from build123d import *

# Parameters (mm, degrees)
BOSS_EXTRUDE1_DEPTH = 7
FILLET1_R           = 3
FILLET2_R           = 5
SKETCH2_W           = 5
SKETCH2_H           = 40
BOSS_EXTRUDE2_DEPTH = 22
SKETCH4_R           = 1.5
CUT_EXTRUDE1_DEPTH  = 3
SKETCH5_R           = 1.5
CUT_EXTRUDE2_DEPTH  = 5
FILLET3_R           = 1


with BuildPart() as part:
    # Sketch1 → Boss-Extrude1 (new body)
    with BuildSketch(Plane(origin=(0, 0, 0), x_dir=(0, 0, -1), z_dir=(1, 0, 0))):
        Polygon((-21.785617828, -17.377868865), (35.214382172, -17.377868865), (35.214382172, 22.622131135), (23.214382172, 22.622131135), (23.214382172, 16.622131135), (1.187686697, 3.773991719), (3.455005417, -0.113072189), (-20.299274017, -13.968908814), (-22.566592737, -10.081844907), (-42.433808264, -21.670362811), (-38.937098948, -27.665079148), align=None)
        Polygon((23.234116709, 8.569586546), (23.234116709, -10.417868865), (4.764740561, -10.417868865), (4.764740561, -1.399885987), (6.011600394, -1.399885987), align=None, mode=Mode.SUBTRACT)
        Polygon((-39.613886954, -22.304550046), (-34.634489281, -19.42911985), (-33.384302239, -21.59407536), (-38.363699913, -24.469505556), align=None, mode=Mode.SUBTRACT)
        Polygon((-9.735540794, -10.497868865), (-2.235259439, -10.497868865), (-2.235259439, -6.248372162), align=None, mode=Mode.SUBTRACT)
        Polygon((16.699385829, 10.182861543), (17.951839541, 8.019216032), (22.7118599, 10.774614335), (21.459406188, 12.938259845), align=None, mode=Mode.SUBTRACT)
    extrude(amount=-BOSS_EXTRUDE1_DEPTH)

    # Fillet1
    # the kernel refuses this fillet: 3 mm, written as the material it adds along each edge
    with BuildSketch(Plane(origin=(0, -10.417868865, -4.764740561), x_dir=(0, 0, -1), z_dir=(-1, 0, 0))) as fillet1_piece_1:
        with BuildLine():
            CenterArc((FILLET1_R, -FILLET1_R), FILLET1_R, 90, 90)
            Line((0, -FILLET1_R), (-FILLET1_R * 0.02, -FILLET1_R))
            Line((-FILLET1_R * 0.02, -FILLET1_R), (-FILLET1_R * 0.02, FILLET1_R * 0.02))
            Line((-FILLET1_R * 0.02, FILLET1_R * 0.02), (FILLET1_R, FILLET1_R * 0.02))
            Line((FILLET1_R, FILLET1_R * 0.02), (FILLET1_R, 0))
        make_face()
    extrude(amount=7)
    with BuildSketch(Plane(origin=(0, -1.399885987, -4.764740561), x_dir=(0, -1, 0), z_dir=(-1, 0, 0))) as fillet1_piece_2:
        with BuildLine():
            CenterArc((2.434440295, -3), FILLET1_R, 90, 54.240794128)
            Line((0, -1.246859832), (-0.048688806, -1.211797029))
            ThreePointArc((-0.048688806, -1.211797029), (-0.06, -0.623429916), (-0.06, 0))
            Line((-0.06, 0), (0, 0.06))
            Line((0, 0.06), (2.434440295, 0.06))
            Line((2.434440295, 0.06), (2.434440295, 0))
        make_face()
    extrude(amount=7)

    # Fillet2
    fillet2_edges = [part.edges().sort_by_distance(p)[0] for p in [
        (-3.5, -10.417868865, -23.234116709),
    ]]
    fillet(fillet2_edges, radius=FILLET2_R)

    # Sketch2 → Boss-Extrude2 (add)
    with BuildSketch(Plane.ZY.offset(7)):
        with Locations((-32.714382172, 2.622131135)):
            Rectangle(SKETCH2_W, SKETCH2_H)
    extrude(amount=BOSS_EXTRUDE2_DEPTH)

    # Sketch4 → Cut-Extrude1 (cut)
    with BuildSketch(Plane(origin=(0, 2.299007828, 1.341007921), x_dir=(1, 0, 0), z_dir=(0, 0.8637919794098133, 0.5038486045502921))):
        with Locations(Location((-3.5, 22.427434704, 0), (0, 0, 270))):
            Circle(SKETCH4_R)
        with Locations(Location((-3.5, -42.572565296, 0), (0, 0, 270))):
            Circle(SKETCH4_R)
    extrude(amount=-CUT_EXTRUDE1_DEPTH, mode=Mode.SUBTRACT)

    # Sketch5 → Cut-Extrude2 (cut)
    with BuildSketch(Plane.XY.offset(-30.214382172)):
        with Locations((-21, 7.622131135)):
            Circle(SKETCH5_R)
        with Locations((-21, -12.377868865)):
            Circle(SKETCH5_R)
    extrude(amount=-CUT_EXTRUDE2_DEPTH, mode=Mode.SUBTRACT)

    # Fillet3
    fillet3_edges = [part.edges().sort_by_distance(p)[0] for p in [
        (-29, 2.622131135, -35.214382172),
        (-29, -17.377868865, -32.714382172),
        (-29, 2.622131135, -30.214382172),
        (-29, 22.622131135, -32.714382172),
    ]]
    fillet(fillet3_edges, radius=FILLET3_R)


solid = part.part
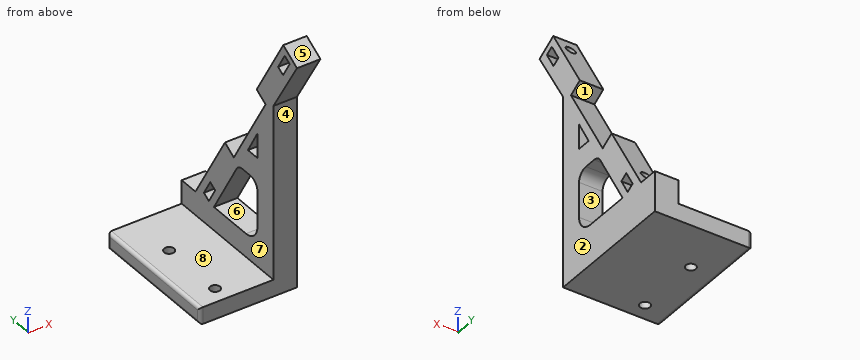
The listing builds one solid part. Answer for the finished solid, in the listing's coordinates (mm). Face numbers are marked on the shaded views. A direction names the side the tool comes from. Coordinates: 2 decimals unless noted, no trailing zeros. Loops run counter-clockwise (first coordinate to the right, second up) from the corner with the lowest first, then second, coordinate; pieces in that order, holes last.
1) Find the intervals of material crossed by L1, parallel to Y at x = -21, z = -33.8; L2, parallel to Y at x = -6.5, z = -17; L3, parallel to Z at x = -9, y = 3, in increasing order.
2) A tool of negligible diameter and unlimited length cuts with its end or side. For the marked faces 1, 2, 3, 4 and 5, from which of +Z, -Z, +X, -X, +Y, -Y can it reach the whole face along a straight path? Write none if from no direction.
3) Determine the mould class of the marked faces 6, 7 and 8 for opening direction Z: pulls with the +Z half, pulls with the -Z half, needs draft (parallel to the pull), parting line crosses it, or undercut.
4) Find section B-B on z = 5. Write down the section's boundary in (x, y).
5) Find section A-A on x = -21. Write down the section's boundary in (y, z).
6) Find section D-D on y = 5. Write down the section's boundary in (x, z).
7) Flat-ended cylindrical pins translate along their axes: pin 1 Ø1.5 at (x, z) = (-8, 14) entering from -Y; pin 2 Ø1.3 at (x, y) = (-4.5, -9) entering from +Z (3 decimals); pin 3 Ø7.5 at (x, z) = (-4, 7.5) entering from +Y; pin 4 Ø1.8 at (x, y) = (-3, 19) entering from +Z. Find the tip coordinate at first contact, or state that the pin passes through.
8) Find section C-C on y = 17.5. Write down the section's boundary in (x, z).
Values:
1. L1: y = -17.38 to -13.88, -10.88 to 6.12, 9.12 to 22.62
1. L2: y = -17.38 to -10.42, 4.96 to 9.66, 10.36 to 13
1. L3: z = -35.21 to -30.21
2. face 1: +X, -X, +Y
2. face 2: +Z, -Z, +X, +Y, -Y
2. face 3: +X, -X
2. face 4: -Z, +X, -X, -Y
2. face 5: +Z, +X, -X, -Y
3. face 6: undercut
3. face 7: needs draft
3. face 8: pulls with the +Z half
4. outline: (-7, -17.38) - (0, -17.38) - (0, -10.5) - (-7, -10.5) - close; (-7, -7.81) - (0, -7.81) - (0, -5.04) - (-7, -5.04) - close
5. outline: (-17.38, -35.21) - (-13.88, -35.21) - (-13.88, -30.21) - (-17.38, -30.21) - close; (-10.88, -35.21) - (6.12, -35.21) - (6.12, -30.21) - (-10.88, -30.21) - close; (9.12, -35.21) - (22.62, -35.21) - (22.62, -30.21) - (9.12, -30.21) - close
6. outline: (-29, -34.21) arc R1 ccw to (-28, -35.21) - (0, -35.21) - (0, -23.23) - (-7, -23.23) - (-7, -30.21) - (-28, -30.21) arc R1 ccw to (-29, -31.21) - close; (-7, -17.07) - (0, -17.07) - (0, -3.29) - (-7, -3.29) - close
7. pin 1: passes through
7. pin 2: stops at z = 12.895
7. pin 3: stops at y = -4.32
7. pin 4: stops at z = -23.21
8. outline: (-29, -34.21) arc R1 ccw to (-28, -35.21) - (0, -35.21) - (0, -23.21) - (-7, -23.21) - (-7, -30.21) - (-28, -30.21) arc R1 ccw to (-29, -31.21) - close
